Autodesk Inventor part; units mm, degrees
ref_plane "YZ Plane" through (0, 0, 0) normal (1, 0, 0) x (0, 1, 0)
ref_plane "XZ Plane" through (0, 0, 0) normal (0, 1, 0) x (-1, 0, 0)
ref_plane "XY Plane" through (0, 0, 0) normal (0, 0, 1) x (1, 0, 0)
sketch "Boceto1" plane through (0, 0, 0) normal (0, 0, 1) x (1, 0, 0)
  line L0 (-7.9599, 1.191) -> (22.0401, 1.191)
  line L1 (22.0401, 1.191) -> (22.0401, -18.809)
  line L2 (22.0401, -18.809) -> (-7.9599, -18.809)
  line L3 (-7.9599, -18.809) -> (-7.9599, 1.191)
  point P0 (0, 0)
  dimension "d0" = 20
  dimension "d10" = 30
extrude "Extrusión1" add sketch "Boceto1" along normal blind 5
sketch "Boceto2" plane through (0, 0, 5) normal (0, 0, 1) x (1, 0, 0)
  line L0 (22.0401, 1.191) -> (22.0401, -18.809)
  line L1 (-7.9599, -18.809) -> (-7.9599, 1.191)
  line L2 (22.0401, -18.809) -> (-7.9599, -18.809)
  circle A0 centre (-5.4599, -8.809) radius 1.75
  circle A1 centre (19.5401, -8.809) radius 1.75
  point P0 (0, 0)
  dimension "d3" = 3.5
  dimension "d4" = 2.5
  dimension "d5" = 2.5
  dimension "d6" = 10
  dimension "d7" = 10
extrude "Extrusión2" cut sketch "Boceto2" against normal blind 5
sketch "Boceto3" plane through (0, 0, 5) normal (0, 0, 1) x (1, 0, 0)
  line L0 (-7.9599, 1.191) -> (22.0401, 1.191)
  line L1 (22.0401, -18.809) -> (-7.9599, -18.809)
  circle A0 centre (7.0401, -3.809) radius 1.75
  circle A1 centre (7.0401, -13.809) radius 1.75
  point P0 (0, 0)
  dimension "d11" = 5
  dimension "d12" = 5
extrude "Extrusión3" cut sketch "Boceto3" against normal blind 5
properties part number "tapa polea x"
Part model, mm, in its own coordinate system. Give positions to 0.01 mm unless a question says otherwise; leave off trailing zeros. Loops run counter-clockwise (first coordinate to the right, second up) from the corner with the lowest first, then second, coordinate; pieces in that order, holes last. Notation, with made-up numbers: M 54.25,43 L 59.25,43 A27 ccw 59.25,73 Z; hole C 43,-23 d5. An arc over 180 degrees is marked long. Put each result on its own line as item: value. Start each with the question number.
1) Probe probe 1 along X at (y, z) = (-8, 2.6); probe 2 along Y at (x, z) = (8.5, 1.2); probe 3 along Y at (x, z) = (19.5, 0.65). List the from-to ranges inside material, lowest first.
2) Saw through at B-B (y = -3.5). List the corners of the cut face in (x, z).
3) Flat gauge pin, fed straight in: pin 1 (12 mm diameter, centred on x = 14, y = -8.5, fed in from -Z). Where does the tip first touch, or does it go through?
4) Pull direction X, two halves, no side cores. Call faces 1 (the cylindrical face through (18.15, -9.87, 2.54)), 2 (the flat face through (7, 1.191, 2)), 3 (the flat face through (22.04, -9, 2)): +X half, -X half, draft (parallel to the pull), parting line (faces both ways), or undercut.
5) Saw through at A-A (z = 3.3). List the corners of the cut face in (x, y).
6) Saw through at C-C (y = -10.25). List the corners of the cut face in (x, z), then the cut area to 3 significant figures.
Numbers:
1. probe 1: -7.96 to -7.01, -3.91 to 17.99, 21.09 to 22.04
1. probe 2: -18.81 to -14.77, -12.84 to -4.77, -2.84 to 1.19
1. probe 3: -18.81 to -10.56, -7.06 to 1.19
2. outline: M -7.96,0 L 5.32,0 L 5.32,5 L -7.96,5 Z; M 8.76,0 L 22.04,0 L 22.04,5 L 8.76,5 Z
3. pin 1: z = 0
4. face 1: undercut
4. face 2: draft
4. face 3: +X half
5. outline: M -7.96,-18.81 L 22.04,-18.81 L 22.04,1.19 L -7.96,1.19 Z; hole C -5.46,-8.81 d3.5; hole C 7.04,-13.81 d3.5; hole C 7.04,-3.81 d3.5; hole C 19.54,-8.81 d3.5
6. outline: M -7.96,0 L -6.45,0 L -6.45,5 L -7.96,5 Z; M -4.47,0 L 18.55,0 L 18.55,5 L -4.47,5 Z; M 20.53,0 L 22.04,0 L 22.04,5 L 20.53,5 Z
6. area: 130 mm^2
